```python
from build123d import *

# Parameters (mm, degrees)
SKETCH1_W           = 70
SKETCH1_H           = 120
BOSS_EXTRUDE1_DEPTH = 3
SKETCH2_R           = 1.75
SKETCH2_R_2         = 3.55
SKETCH2_W           = 28
SKETCH2_H           = 16
CUT_EXTRUDE1_DEPTH  = 3
SKETCH4_R           = 3.55
CUT_EXTRUDE2_DEPTH  = 12


with BuildPart() as part:
    # Sketch1 → Boss-Extrude1 (new body)
    with BuildSketch(Plane(origin=(0, 0, 0), x_dir=(1, 0, 0), z_dir=(0, 1, 0))):
        with Locations((35, 60)):
            Rectangle(SKETCH1_W, SKETCH1_H)
    extrude(amount=BOSS_EXTRUDE1_DEPTH)

    # Sketch2 → Cut-Extrude1 (cut)
    with BuildSketch(Plane(origin=(0, 3, 0), x_dir=(1, 0, 0), z_dir=(0, 1, 0))):
        with Locations(Location((11, 92, 0), (0, 0, 270))):
            Circle(SKETCH2_R)
        with Locations(Location((59, 92, 0), (0, 0, 270))):
            Circle(SKETCH2_R)
        with Locations(Location((52.5, 24, 0), (0, 0, 270))):
            Circle(SKETCH2_R_2)
        with Locations(Location((17.5, 24, 0), (0, 0, 270))):
            Circle(SKETCH2_R_2)
        with Locations(Location((7, 113, 0), (0, 0, 270))):
            Circle(SKETCH2_R)
        with Locations(Location((63, 113, 0), (0, 0, 270))):
            Circle(SKETCH2_R)
        with Locations(Location((63, 7, 0), (0, 0, 270))):
            Circle(SKETCH2_R)
        with Locations(Location((7, 7, 0), (0, 0, 270))):
            Circle(SKETCH2_R)
        with Locations((35, 92)):
            Rectangle(SKETCH2_W, SKETCH2_H)
    extrude(amount=-CUT_EXTRUDE1_DEPTH, mode=Mode.SUBTRACT)

    # Sketch4 → Cut-Extrude2 (cut)
    with BuildSketch(Plane(origin=(0, 3, 0), x_dir=(1, 0, 0), z_dir=(0, 1, 0))):
        with Locations(Location((17.5, 50, 0), (0, 0, 270))):
            Circle(SKETCH4_R)
        with Locations(Location((52.5, 50, 0), (0, 0, 270))):
            Circle(SKETCH4_R)
    extrude(amount=-CUT_EXTRUDE2_DEPTH, mode=Mode.SUBTRACT)


solid = part.part
```
Build history of the part. All positions in model axes, mm. A direction names the side the tool comes from. Round coordinates to 2 decimals unless told otherwise and drop trailing zeros. Loops run counter-clockwise (first coordinate to the right, second up) from the corner with the lowest first, then second, coordinate; pieces in that order, holes last.
Item 1: Two-plate mould, pull along Z, no slides. Class faces 3 (the face through (19.899, 1.521, -26.616)), 4 (the face through (35, 3, -61)), 5 (the face through (5.29, 1.52, -113.38)), 6 (the face through (35, 1, 0)): released by +Z, released by -Z, zero draft, split by the parting line, or undercut.
Item 2: Saw through at D-D (z = -24). List the corners of the cut face in (x, y), then the cut area to 3 significant figures.
Item 3: Saw through at A-A (x = 11). List the corners of the cut face in (y, z).
Item 4: Saw through at B-B (z = -92). List the corners of the cut face in (x, y).
Item 5: Pin check, flat tip, straight feed: P1, Ø1.5, axis at x = 61, y = 2.5, coming from the +Z side. Stop position of the tip, or through.
Item 6: Saw through at C-C (y = 0.9). State how many separate pieces and enclosed holes the cut face has, then the cut area to 3 significant figures.
Item 7: Drill centre lines: line 1 along X through (y, z) = (1.8, -92); line 2 along X through (y, z) = (0.7, -113); line 3 along X through (y, z) = (1.7, -50). Where is each one in solid material? Low to high.
Item 8: Which spindle directions (+Z, -Z, +X, -X, +Y, -Y) get a long thin tool onto all of the face, cutting with end or side? Do faces 1 (the face through (35, 1, -120)), 2 (the face through (35, 2, -100)). Say none if no direction does.
Worked answers:
1. face 3: undercut
1. face 4: zero draft
1. face 5: undercut
1. face 6: released by +Z
2. outline: (0, 0) - (13.95, 0) - (13.95, 3) - (0, 3) - close; (21.05, 0) - (48.95, 0) - (48.95, 3) - (21.05, 3) - close; (56.05, 0) - (70, 0) - (70, 3) - (56.05, 3) - close
2. area: 167 mm2
3. outline: (0, -120) - (3, -120) - (3, -93.75) - (0, -93.75) - close; (0, -90.25) - (3, -90.25) - (3, 0) - (0, 0) - close
4. outline: (0, 0) - (9.25, 0) - (9.25, 3) - (0, 3) - close; (12.75, 0) - (21, 0) - (21, 3) - (12.75, 3) - close; (49, 0) - (57.25, 0) - (57.25, 3) - (49, 3) - close; (60.75, 0) - (70, 0) - (70, 3) - (60.75, 3) - close
5. P1: stops at z = 0
6. separate pieces: 1
6. enclosed holes: 11
6. area: 7,740 mm2
7. line 1: x = 0 to 9.25, 12.75 to 21, 49 to 57.25, 60.75 to 70
7. line 2: x = 0 to 5.25, 8.75 to 61.25, 64.75 to 70
7. line 3: x = 0 to 13.95, 21.05 to 48.95, 56.05 to 70
8. face 1: -Z, +X, -X, +Y, -Y
8. face 2: +Y, -Y
